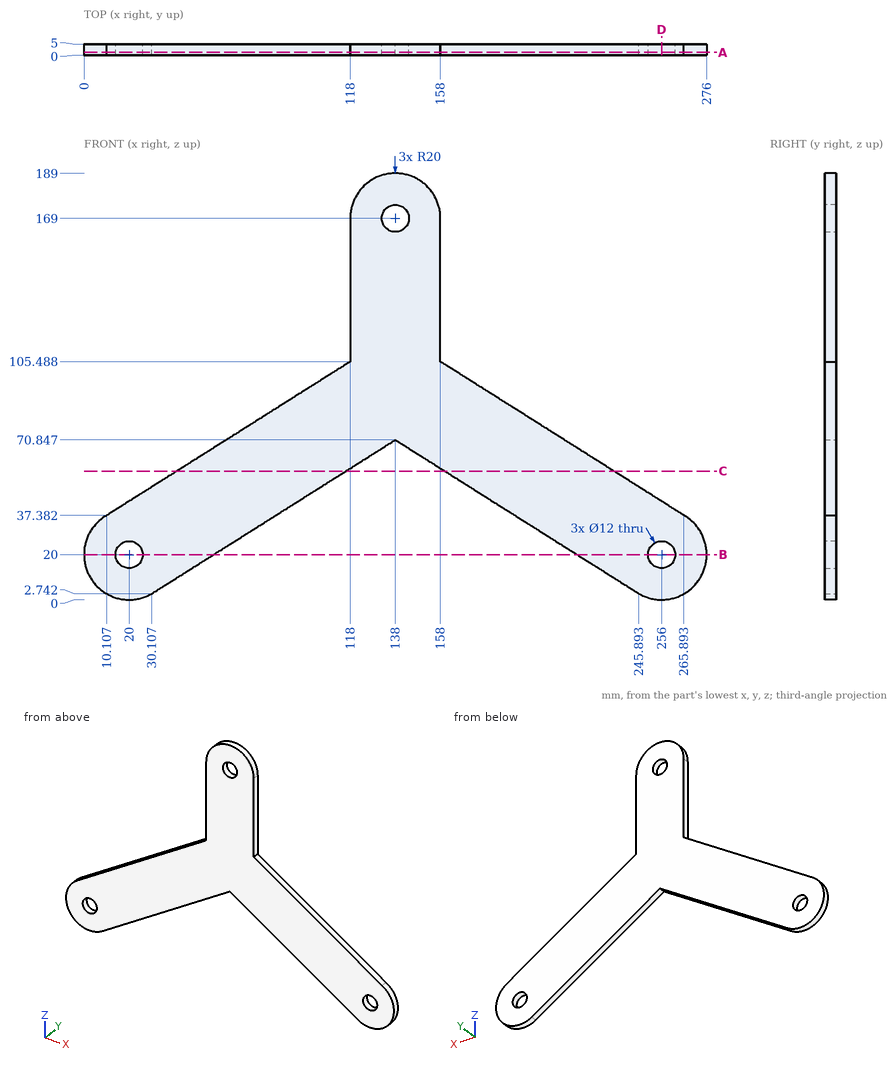
Input: dimensioned drawing with shaded views. Units: mm. Origin: part minimum x, y, z. Round coordinates to 2 decimals unless told otherwise and drop trailing zeros. Order: outer loops, then holes, each group sorted by start corner. A loop starts at its lowest first (then second) coordinate and runs counter-clockwise, first axis right, second up. Notation, with made-up numbers: M -21,-26.5 L 15,-26.5 A22 ccw 15,-8.5 Z; hole C 61,-29 d7. An arc over 180 degrees is marked long. Use one line per item in the form item = value. Start each with the question number.
Q1. Cut plane A-A (y = 1.25). Return loops of the section in (x, z).
Q2. Cut plane D-D (x = 256). Return loops of the section in (y, z).
Q3. Material intervals for line 1 (Z direction, x = 138, y = 1.55); line 2 (X direction, y = 2.4, z = 169); line 3 (X direction, y = 3.55, z = 162.5), sorted ascending. Write a range as [from, to].
Q4. Cut plane C-C (z = 57). Return loops of the section in (x, y).
Q5. Pin query (flat end, axial travel): pin 1 Ø1.5 at (y, z) = (2, 137.5) entering from +X; pin 2 Ø1.5 at (x, y) = (180.5, 3.5) entering from -Z; pin 3 Ø2 at (x, y) = (145, 2.5) entering from +Z. Return the tip coordinate at first contact, or that it passes through.
Q6. Cut plane B-B (z = 20). Return loops of the section in (x, y).
Geometry results:
q1.outline = M 10.11,37.38 A20 ccw long 30.11,2.74 L 138,70.85 L 245.89,2.74 A20 ccw long 265.89,37.38 L 158,105.49 L 158,168.97 A20 ccw 118,168.97 L 118,105.49 Z; hole C 20,20 d12; hole C 138,169 d12; hole C 256,20 d12
q2.outline = M 0,0 L 5,0 L 5,14 L 0,14 Z; M 0,26 L 5,26 L 5,43.63 L 0,43.63 Z
q3.line_1 = [70.85, 163], [175, 189]
q3.line_2 = [118, 132], [144, 158]
q3.line_3 = [118, 158]
q4.outline = M 41.19,0 L 116.06,0 L 116.06,5 L 41.19,5 Z; M 159.94,0 L 234.81,0 L 234.81,5 L 159.94,5 Z
q5.pin_1 = 158
q5.pin_2 = 43.55
q5.pin_3 = 188.08
q6.outline = M 0,0 L 14,0 L 14,5 L 0,5 Z; M 26,0 L 57.45,0 L 57.45,5 L 26,5 Z; M 218.55,0 L 250,0 L 250,5 L 218.55,5 Z; M 262,0 L 276,0 L 276,5 L 262,5 Z
